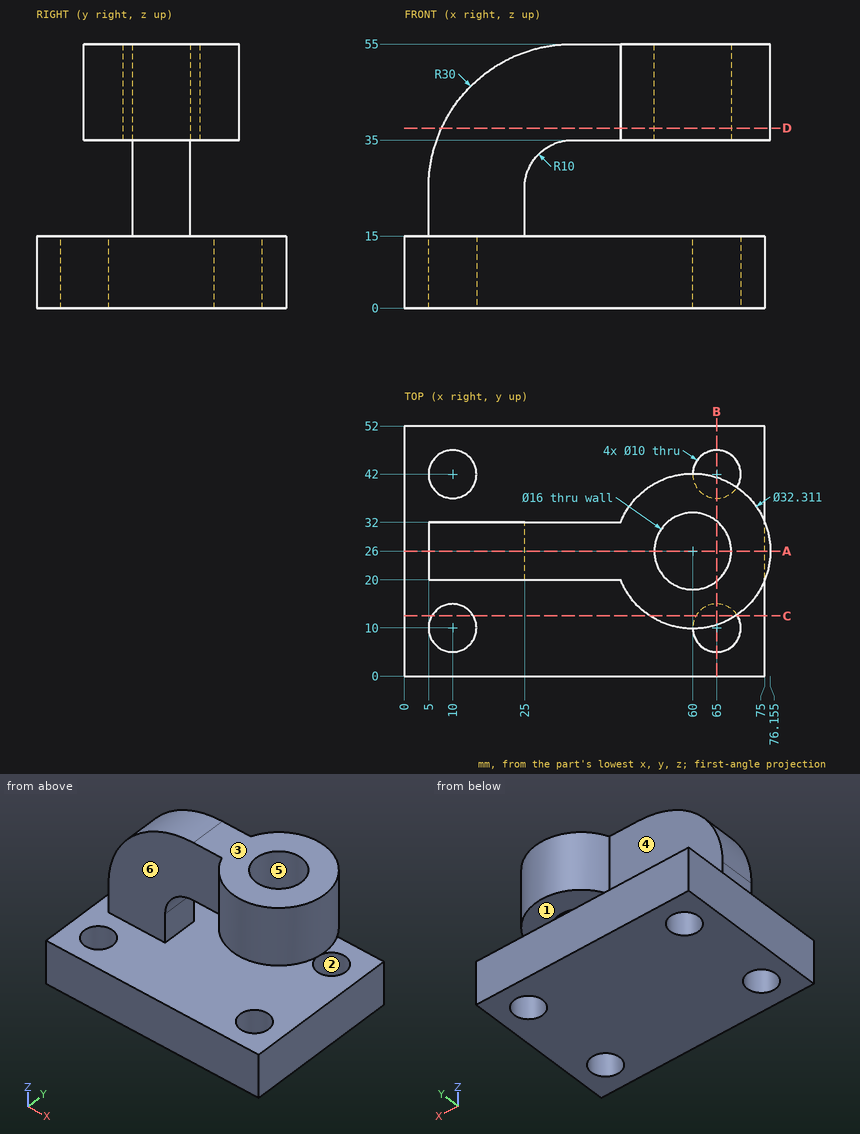
Here's the drawing with two shaded views (mm, measured from the low corner). I have some questions. A direction names the side the tool comes from. Coordinates: 2 decimals unless noted, no trailing zeros. Loops run counter-clockwise (first coordinate to the right, second up) from the corner with the lowest first, then second, coordinate; pieces in that order, holes last. Notation, with made-up numbers: M 88.25,10.5 L 107.25,10.5 A22 cw 107.25,26.5 Z; hole C -4.5,7 d10. An arc over 180 degrees is marked long. Return JSON: item names as keys, results as strings. Group by question number.
Item 1: If I drill on L1, parallel to Y at x = 65, z = 3; L2, parallel to X at y = 7, z = 12.5; L3, parallel to Y at x = 60, z = 44 (1 decimal), over which ranges is the centre line in solid material (lowest first)? Write a range as from..to.
Item 2: Imagine slicing it at C-C (y = 12.5). Please give me the cut outline in (x, z) (1 decimal), and give its area (3 significant figures).
Item 3: Imagine slicing it at D-D (z = 37.5). Please give me the cut outline in (x, y) (1 decimal), and give its area (3 significant figures).
Item 4: Imagine slicing it at A-A (y = 26). Please give me the cut outline in (x, z) (1 decimal), and give its area (3 significant figures).
Item 5: On a 3-axis mill with a long thin cutter (end or side, diameter ignored), from which of +Z, -Z, +X, -X, +Y, -Y can I reach the whole of each face in a straight line? I mean the marked faces 4, 5 and 6. Say none if no direction works.
Item 6: Imagine slicing it at B-B (x = 65). Please give me the cut outline in (y, z) (1 decimal).
Item 7: I'm going to push flat-ended pins straight in: pin 1 Ø12 at (x, z) = (15, 33.5) entering from +Y; pin 2 Ø3 at (y, z) = (23.5, 12.5) entering from +X; pin 3 Ø14.5 at (x, y) = (60, 26) entering from +Z. Where does each tip first touch, or does it pass through?
Item 8: Thinking about a two-plate mould opening in Z: for the marked faces 1, 2 and 3, which applies, released by +Z, released by -Z, zero draft, split by the parting line, or undercut?
Verdict:
{
 "1": {"L1": "y = 0..5, 15..37, 47..52", "L2": "x = 0..6, 14..61, 69..75", "L3": "y = 9.8..18, 34..42.2"},
 "2": {"outline": "M 0,0 L 5.7,0 L 5.7,15 L 0,15 Z; M 14.3,0 L 60.7,0 L 60.7,15 L 14.3,15 Z; M 51.1,35 L 68.9,35 L 68.9,55 L 51.1,55 Z; M 69.3,0 L 75,0 L 75,15 L 69.3,15 Z", "area": "1,220 mm^2"},
 "3": {"outline": "M 7.7,20 L 45,20 A16.2 ccw long 45,32 L 7.7,32 Z; hole C 60,26 d16", "area": "1,060 mm^2"},
 "4": {"outline": "M 0,0 L 75,0 L 75,15 L 25,15 L 25,25 A10 cw 35,35 L 52,35 L 52,55 L 35,55 A30 ccw 5,25 L 5,15 L 0,15 Z; M 68,35 L 76.2,35 L 76.2,55 L 68,55 Z", "area": "2,460 mm^2"},
 "5": {"face 4": "+Z, -X, +Y", "face 5": "+Z", "face 6": "+Z, -X, -Y"},
 "6": {"outline": "M 0,0 L 5,0 L 5,15 L 0,15 Z; M 10.6,35 L 19.8,35 L 19.8,55 L 10.6,55 Z; M 15,0 L 37,0 L 37,15 L 15,15 Z; M 32.2,35 L 41.4,35 L 41.4,55 L 32.2,55 Z; M 47,0 L 52,0 L 52,15 L 47,15 Z"},
 "7": {"pin 1": "stops at y = 32", "pin 2": "stops at x = 75", "pin 3": "stops at z = 15"},
 "8": {"face 1": "undercut", "face 2": "zero draft", "face 3": "released by +Z"}
}
